```python
from build123d import *

# Parameters (mm, degrees)
SKETCH037_R   = 49
SKETCH037_R_2 = 27.5
PAD028_DEPTH  = 67
SKETCH035_R   = 100
SKETCH035_R_2 = 27
PAD026_DEPTH  = 3.5
SKETCH036_R   = 100
SKETCH036_R_2 = 27
PAD027_DEPTH  = 3.5


with BuildPart() as part:
    # Sketch037 → Pad028 (new body)
    with BuildSketch(Plane.XY):
        Circle(SKETCH037_R)
        Circle(SKETCH037_R_2, mode=Mode.SUBTRACT)
    extrude(amount=PAD028_DEPTH)

    # Sketch035 → Pad026 (join)
    with BuildSketch(Plane.XY):
        Circle(SKETCH035_R)
        Circle(SKETCH035_R_2, mode=Mode.SUBTRACT)
    extrude(amount=PAD026_DEPTH)

    # Sketch036 → Pad027 (join)
    with BuildSketch(Plane.XY.offset(67)):
        Circle(SKETCH036_R)
        Circle(SKETCH036_R_2, mode=Mode.SUBTRACT)
    extrude(amount=-PAD027_DEPTH)


with BuildPart() as part_1:
    # Body008 placement: moved
    add(part.part.moved(Location((0, 0, 63))))


solid = part_1.part
```
Model file for the job. Use its own axes, mm. A direction names the side the tool comes from. Round coordinates to 2 decimals unless told otherwise and drop trailing zeros. Write each loop counter-clockwise with the first axis right and the second up, starting at its lowest first coordinate (ties: lowest second). Pieces come first, ordered by that corner, then holes. Notation, with made-up numbers: (63, 80) -> (118, 80) arc R29 cw to (118, 108) -> close; hole circle Ø3 at (8, -13). An arc over 180 degrees is marked (long way). Answer as CSV lines item,"result".
1. Mould opens along X. For faces 1 (the face through (-5.961, -26.846, 96.08)), 2 (the face through (26.34, 41.32, 96.08)), 3 (the face through (20.2, -18.2, 126.5)), 4 (the face through (-24, -43, 66.5)) say: +X half, -X half, draft (parallel to the pull), parting line (faces both ways), or undercut.
Resolved:
face 1,"undercut"
face 2,"parting line"
face 3,"undercut"
face 4,"draft"
2. Pin check, flat tips, straight feed: pin 1 Ø4 at (y, z) = (-31.5, 75) entering from -X; pin 2 Ø2 at (y, z) = (17.5, 115) entering from +X; pin 3 Ø8 at (x, z) = (-23, 106) entering from -Y. Stop position of each tip, or through.
Resolved:
pin 1,"x = -39.12"
pin 2,"x = 46.14"
pin 3,"y = -45.17"
3. Tool access for faces 5 (the face through (20.2, -18.2, 66.5)), 6 (the face through (95.38, 30.04, 64.73)): list every direction of +Z, -Z, +X, -X, +Y, -Y with a clear straight run to the whole face (end or side of a thin tool).
Resolved:
face 5,"none"
face 6,"+Z, -Z"
4. Slice it at C-C, the plane z = 88.5. List the corners of the cut face in (x, y).
Resolved:
outline,"circle Ø98 at (0, 0); hole circle Ø55 at (0, 0)"
5. Slice it at D-D, the plane y = -75. List the corners of the cut face in (x, z), plus the area to 3 significant figures.
Resolved:
outline,"(-66.14, 63) -> (66.14, 63) -> (66.14, 66.5) -> (-66.14, 66.5) -> close; (-66.14, 126.5) -> (66.14, 126.5) -> (66.14, 130) -> (-66.14, 130) -> close"
area,"926 mm²"
6. Slice it at A-A, the plane x = 0. List the corners of the cut face in (y, z), plus the area to 3 significant figures.
Resolved:
outline,"(-100, 63) -> (-27, 63) -> (-27, 66.5) -> (-27.5, 66.5) -> (-27.5, 126.5) -> (-27, 126.5) -> (-27, 130) -> (-100, 130) -> (-100, 126.5) -> (-49, 126.5) -> (-49, 66.5) -> (-100, 66.5) -> close; (27, 63) -> (100, 63) -> (100, 66.5) -> (49, 66.5) -> (49, 126.5) -> (100, 126.5) -> (100, 130) -> (27, 130) -> (27, 126.5) -> (27.5, 126.5) -> (27.5, 66.5) -> (27, 66.5) -> close"
area,"3,600 mm²"
7. Drill centre lines: line 1 (Z direction, x = 33.5, y = 38); line 2 (Y direction, x = 0, z = 79). Where is each one in solid material? Low to high.
Resolved:
line 1,"63 to 66.5, 126.5 to 130"
line 2,"-49 to -27.5, 27.5 to 49"
